Part model, mm, in its own coordinate system. Coordinates: 2 decimals unless noted, no trailing zeros. Write each loop counter-clockwise with the first axis right and the second up, starting at its lowest first coordinate (ties: lowest second). Pieces come first, ordered by that corner, then holes. Notation, with made-up numbers: (-36, 44) -> (-13, 44) arc R25 ccw to (-13, 58) -> close; hole circle Ø6 at (75.5, 57). An arc over 180 degrees is marked (long way). Write item = value, one per line. Start each with the question number.
Q1. Band-saw the part on B-B, the plane x = -2.5. List the corners of the cut face in (y, z), plus the area to 3 significant figures.
Q2. Probe line 1 (Z direction, x = 0, y = 0.45); line 2 (X direction, y = 0.15, z = 39.5); line 3 (X direction, y = 0.6, z = -8). List the from-to ranges inside material, lowest first.
Q3. Band-saw the part on C-C, the plane y = 0.8. List the corners of the cut face in (x, z).
Q4. Pin check, flat tip, straight feed: P1, Ø10, axis at x = 23.5, z = 35.5, coming from the +Y side. Stop position of the tip, or through.
Q5. Band-saw the part on A-A, the plane z = 0. List the corners of the cut face in (x, y), plus the area to 3 significant figures.
Q6. Pull direction X, two halves, no side cores. Call faces 1 (the cylindrical face through (-52.654, 0.493, 21.831)), 2 (the cylindrical face through (-47.954, 0.507, -2.11)), 3 (the flat face through (30, 0, -38)): released by +X, released by -X, zero draft, split by the parting line, or undercut.
Autodesk Inventor part; units mm, degrees
ref_plane "YZ Plane" through (0, 0, 0) normal (1, 0, 0) x (0, 1, 0)
ref_plane "XZ Plane" through (0, 0, 0) normal (0, 1, 0) x (-1, 0, 0)
ref_plane "XY Plane" through (0, 0, 0) normal (0, 0, 1) x (1, 0, 0)
sketch "Skizze5" plane through (0, 0, 0) normal (0, 0, 1) x (1, 0, 0)
  line L0 (0, 0) -> (0, -48)
  arc A0 (-48, 0) -> (0, -48) centre (0, 0) ccw
  dimension "d17" = 48
surface revolve "Rotationsfläche3" sketch "Skizze5" angle 360 about axis through (0, 0, 0) along (0, -1, 0) shown yes curves A0 L0
sketch "Skizze6" plane through (0, 0, 0) normal (0, 0, 1) x (1, 0, 0)
  line L0 (0, 0) -> (0, -49)
  arc A0 (-49, 0) -> (0, -49) centre (0, 0) ccw
  dimension "d19" = 49
surface revolve "Rotationsfläche4" sketch "Skizze6" angle 360 about axis through (0, 0, 0) along (0, -1, 0) shown yes curves A0 L0
sketch "Skizze7" plane through (0, 0, 0) normal (0, 1, 0) x (-1, 0, 0)
  circle A0 centre (0, 0) radius 57
  dimension "d21" = 114
extrude "Extrusion1" add sketch "Skizze7" along normal blind 1
sketch "Skizze8" plane through (0, 1, 0) normal (0, 1, 0) x (1, 0, 0)
  point P0 (0, 0)
sketch "Skizze9" plane through (0, 1, 0) normal (0, 1, 0) x (1, 0, 0)
  circle A0 centre (0, 0) radius 48
extrude "Extrusion2" cut sketch "Skizze9" against normal blind 1
properties part number "Futterschüssel_innen" material "Edelstahl"
Ans:
q1.outline = (0, -56.95) -> (1, -56.95) -> (1, -47.93) -> (0, -47.93) -> close; (0, 47.93) -> (1, 47.93) -> (1, 56.95) -> (0, 56.95) -> close
q1.area = 18.0 mm2
q2.line_1 = -57 to -48, 48 to 57
q2.line_2 = -41.09 to -27.27, 27.27 to 41.09
q2.line_3 = -56.44 to -47.33, 47.33 to 56.44
q3.outline = circle Ø114 at (0, 0); hole circle Ø96 at (0, 0)
q4.P1 = through
q5.outline = (-57, 0) -> (-48, 0) -> (-48, 1) -> (-57, 1) -> close; (48, 0) -> (57, 0) -> (57, 1) -> (48, 1) -> close
q5.area = 18.0 mm2
q6.face_1 = split by the parting line
q6.face_2 = undercut
q6.face_3 = zero draft
